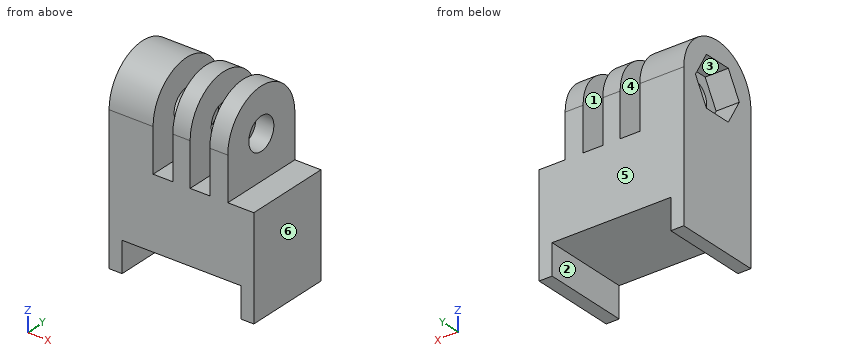
```python
from build123d import *

# Parameters (mm, degrees)
SKETCH009_R     = 2.8
PAD_DEPTH       = 12.5
SKETCH015_W     = 20.5
SKETCH015_H     = 10.5
SKETCH015_W_2   = 3.4
SKETCH015_H_2   = 15
SKETCH015_W_3   = 15
POCKET_DEPTH    = 15
POCKET001_DEPTH = 4


with BuildPart() as part:
    # Sketch009 → Pad (new body, symmetric)
    with BuildSketch(Plane.YZ):
        with BuildLine():
            Line((7.5, 25), (7.5, 0))
            Line((-7.5, 0), (7.5, 0))
            Line((-7.5, 0), (-7.5, 25))
            ThreePointArc((7.5, 25), (0, 32.5), (-7.5, 25))
        make_face()
        with Locations((0, 25)):
            Circle(SKETCH009_R, mode=Mode.SUBTRACT)
    extrude(amount=PAD_DEPTH, both=True)

    # Sketch015 → Pocket (cut, symmetric)
    with BuildSketch(Plane.XZ):
        Rectangle(SKETCH015_W, SKETCH015_H)
        with Locations((3.2, 25)):
            Rectangle(SKETCH015_W_2, SKETCH015_H_2)
        with Locations((15.5, 25)):
            Rectangle(SKETCH015_W_3, SKETCH015_H_2)
        with Locations((-3.2, 25)):
            Rectangle(SKETCH015_W_2, SKETCH015_H_2)
    extrude(amount=POCKET_DEPTH, both=True, mode=Mode.SUBTRACT)

    # Sketch016 → Pocket001 (cut)
    with BuildSketch(Plane.YZ.offset(-12.5)):
        Polygon((-2.45, 20.756476), (2.45, 20.756476), (4.9, 25), (2.45, 29.243524), (-2.45, 29.243524), (-4.9, 25), align=None)
    extrude(amount=POCKET001_DEPTH, mode=Mode.SUBTRACT)


solid = part.part
```
Can you work these out from the model? Positions are in its coordinate system, mm. Face numbers are marked on the shaded views. A direction names the side the tool comes from. Coordinates: 2 decimals unless noted, no trailing zeros. Write each loop counter-clockwise with the first axis right and the second up, starting at its lowest first coordinate (ties: lowest second). Pieces come first, ordered by that corner, then holes. Notation, with made-up numbers: M -24.5,19 L 18.5,19 A14 ccw 18.5,40 Z; hole C 78,86 d2. An arc over 180 degrees is marked long. Write item = value, one per line. Start each with the question number.
Q1. If we section it at C-C, the plane x = 3: Write out the boundary of the cut face in (y, z).
Q2. On a 3-axis mill with a long thin cutter (end or side, diameter ignored), from which of +Z, -Z, +X, -X, +Y, -Y can I reach the whole of each face in a straight line? I mean the marked faces 1, 2 and 3. Say none if no direction works.
Q3. If we section it at A-A, the plane y = 0: State how many separate pieces and enclosed holes the cut face has, then the cut area to 3 significant figures.
Q4. If we section it at D-D, the plane y = -4: Write out the boundary of the cut face in (x, z), then the cut area to 3 significant figures.
Q5. Thinking about a two-plate mould opening in X: for the marked faces 4, 5 and 6, which applies, released by +X, released by -X, zero draft, split by the parting line, or undercut?
Q6. If we section it at B-B, the plane y = -6: Write out the boundary of the cut face in (x, z).
Q7. If I drill on L1, parallel to X at y = 3.75, z = 22; L2, parallel to Y at x = 7.3, z = 25; L3, parallel to X at y = 2.5, z = 3, over which ranges is the centre line in solid material (lowest first)? Write a range as [from, to].
Q8. I'm going to push flat-ended pins straight in: pin 1 (2 mm diameter, centred on x = 10.5, y = -1.5, fed in from +Z); pin 2 (9 mm diameter, centred on y = 0, z = 25, fed in from +X); pin 3 (5 mm diameter, centred on x = -4, y = -6, fed in from +Z); pin 4 (5 mm diameter, centred on y = 0, z = 25, fed in from +X). Where does each tip first touch, or does it pass through?
Check sheet entries:
q1.outline = M -7.5,5.25 L 7.5,5.25 L 7.5,17.5 L -7.5,17.5 Z
q2.face_1 = +Z, +Y, -Y
q2.face_2 = -Z, +Y, -Y
q2.face_3 = -X
q3.separate_pieces = 4
q3.enclosed_holes = 0
q3.area = 447 mm²
q4.outline = M -12.5,0 L -10.25,0 L -10.25,5.25 L 10.25,5.25 L 10.25,0 L 12.5,0 L 12.5,17.5 L 8,17.5 L 8,31.34 L 4.9,31.34 L 4.9,17.5 L 1.5,17.5 L 1.5,31.34 L -1.5,31.34 L -1.5,17.5 L -4.9,17.5 L -4.9,31.34 L -12.5,31.34 L -12.5,26.56 L -8.5,26.56 L -8.5,23.44 L -12.5,23.44 Z
q4.area = 507 mm²
q5.face_4 = undercut
q5.face_5 = zero draft
q5.face_6 = released by +X
q6.outline = M -12.5,0 L -10.25,0 L -10.25,5.25 L 10.25,5.25 L 10.25,0 L 12.5,0 L 12.5,17.5 L 8,17.5 L 8,29.5 L 4.9,29.5 L 4.9,17.5 L 1.5,17.5 L 1.5,29.5 L -1.5,29.5 L -1.5,17.5 L -4.9,17.5 L -4.9,29.5 L -12.5,29.5 Z
q7.L1 = [-12.5, -4.9], [-1.5, 1.5], [4.9, 8]
q7.L2 = [-7.5, -2.8], [2.8, 7.5]
q7.L3 = [-12.5, -10.25], [10.25, 12.5]
q8.pin_1 = 17.5
q8.pin_2 = 8
q8.pin_3 = 31.54
q8.pin_4 = through
